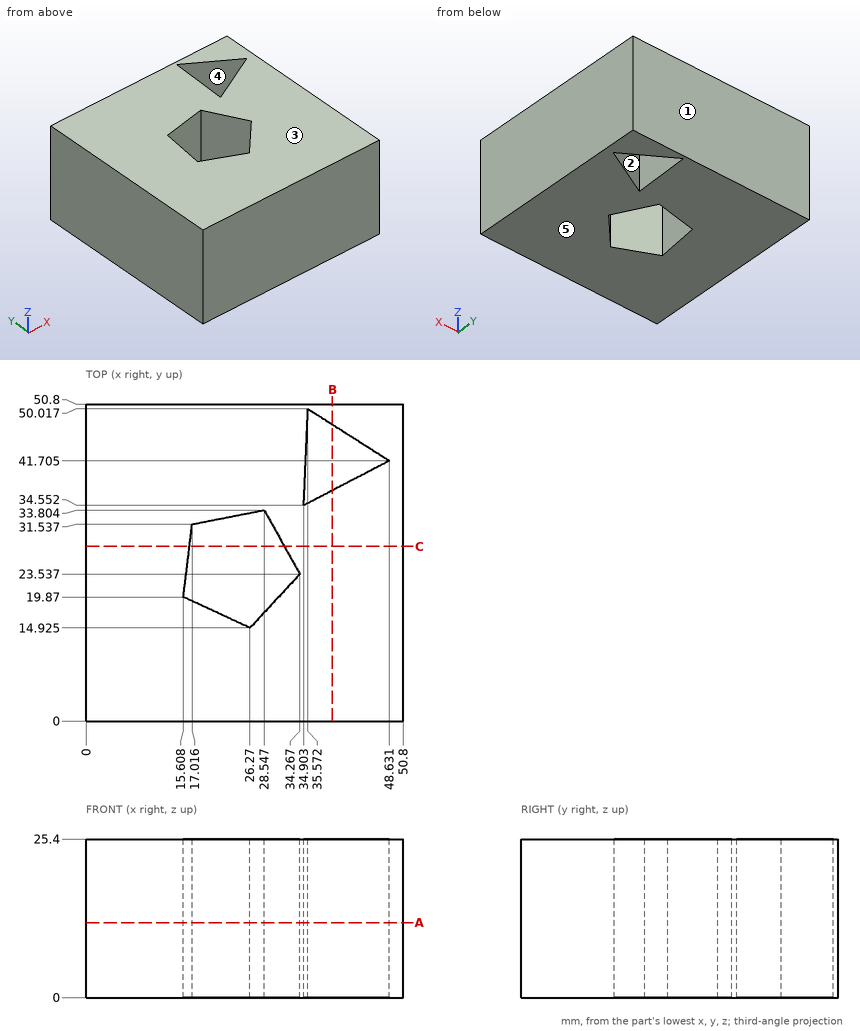
Check sheet for the drawn part. Datum: minimum x, y, z corner. Units: mm. A direction names the side the tool comes from. Give positions to 0.01 mm unless a question says otherwise; leave off trailing zeros. Order: outer loops, then holes, each group sorted by start corner. A loop starts at its lowest first (then second) coordinate and runs counter-clockwise, first axis right, second up. Notation, with made-up numbers: (28.25, 50.5) - (65.25, 50.5) arc R15 ccw to (65.25, 78.5) - close; hole circle Ø1 at (45, 58). An arc over 180 degrees is marked (long way). Answer in a Markdown table with one row per item. Add a question column.
Q1. Mould release check, pull along Y, two halves, no side actions. Record for the marked faces 1, 2 and 3: pulls with the +Y half, pulls with the -Y half, needs draft (parallel to the pull), parting line crosses it, or undercut.
Q2. Material ranges on probe 1 along X at (y, z) = (23.5, 15) (1 decimal); probe 2 along Y at (x, z) = (32, 16.5) (1 decimal); probe 3 along Y at (x, z) = (47.5, 13.75) (1 decimal), recorded low to high. Write a range as from..to.
Q3. Tool access check on the marked faces 4 and 5. Record the directions out of +Z, -Z, +X, -X, +Y, -Y that give a thin tool (end or side, any length) a straight path to the whole face; none if there is none.
Q4. Cross-section at A-A, the plane z = 12. Enter the section's corners in (x, y) (1 decimal).
Q5. Cross-section at B-B, the plane x = 39.5. Enter the section's corners in (y, z), then the cut area to 3 significant figures.
Q6. Cross-section at C-C, the plane y = 28. Enter the section's corners in (x, z).
Q7. Gauge pin test, flat end, axial feed: pin 1 (4 mm diameter, centred on x = 19.5, y = 28.5, fed in from -Z). Record the tip position at first contact, or that the pin passes through.
Check values:
| question | item | result |
|---|---|---|
| 1 | face 1 | pulls with the +Y half |
| 1 | face 2 | undercut |
| 1 | face 3 | needs draft |
| 2 | probe 1 | x = 0..16, 34.2..50.8 |
| 2 | probe 2 | y = 0..21.1, 27.6..50.8 |
| 2 | probe 3 | y = 0..41.1, 42.4..50.8 |
| 3 | face 4 | +Z, -Z |
| 3 | face 5 | -Z, +X, -X, +Y, -Y |
| 4 | outline | (0, 0) - (50.8, 0) - (50.8, 50.8) - (0, 50.8) - close; hole (15.6, 19.9) - (26.3, 14.9) - (34.3, 23.5) - (28.5, 33.8) - (17, 31.5) - close; hole (34.9, 34.6) - (48.6, 41.7) - (35.6, 50) - close |
| 5 | outline | (0, 0) - (36.95, 0) - (36.95, 25.4) - (0, 25.4) - close; (47.52, 0) - (50.8, 0) - (50.8, 25.4) - (47.52, 25.4) - close |
| 5 | area | 1,020 mm^2 |
| 6 | outline | (0, 0) - (16.59, 0) - (16.59, 25.4) - (0, 25.4) - close; (31.78, 0) - (50.8, 0) - (50.8, 25.4) - (31.78, 25.4) - close |
| 7 | pin 1 | passes through |
